Autodesk Inventor part; units mm, degrees
ref_plane "YZ Plane" through (0, 0, 0) normal (1, 0, 0) x (0, 1, 0)
ref_plane "XZ Plane" through (0, 0, 0) normal (0, 1, 0) x (-1, 0, 0)
ref_plane "XY Plane" through (0, 0, 0) normal (0, 0, 1) x (1, 0, 0)
sketch "Sketch1" plane through (0, 0, 0) normal (0, 1, 0) x (-1, 0, 0)
  line L0 (-175, 175) -> (-175, -175)
  line L1 (-175, -175) -> (175, -175)
  line L2 (175, -175) -> (175, 175)
  line L3 (175, 175) -> (-175, 175)
  line L4 (-175, 175) -> (175, -175) construction
  line L5 (-175, -175) -> (175, 175) construction
  point P0 (0, 0)
  dimension "d0" = 350
  dimension "d1" = 350
extrude "Extrusion1" add sketch "Sketch1" along normal blind 10
sketch "Sketch2" plane through (0, 10, 0) normal (0, 1, 0) x (1, 0, 0)
  line L0 (175, -175) -> (175, 175)
  line L1 (175, 175) -> (-175, 175)
  line L2 (-175, 175) -> (-175, -175)
  line L3 (-175, -175) -> (175, -175)
  line L4 (-175, 175) -> (175, -175) construction
  line L5 (-175, -175) -> (175, -175) construction
  line L6 (-175, -175) -> (161.7326, 161.7326) construction
  line L7 (40, -40) -> (40, 40)
  line L8 (40, 40) -> (-40, 40)
  line L9 (-40, 40) -> (-40, -40)
  line L10 (-40, -40) -> (40, -40)
  line L11 (40, -40) -> (-40, 40) construction
  line L12 (40, 40) -> (-40, -40) construction
  point P0 (0, 0)
  dimension "d4" = 80
  dimension "d5" = 80
extrude "Extrusion2" cut sketch "Sketch2" against normal blind 10 contours L10 L9 L8 L7
sketch "Sketch3" plane through (0, 10, 0) normal (0, 1, 0) x (1, 0, 0)
  line L0 (40, -40) -> (-40, -40)
  point P0 (0, 0)
sketch "Sketch4" plane through (0, 10, 0) normal (0, 1, 0) x (1, 0, 0)
  line L0 (40, -40) -> (-40, -40) construction
  line L1 (45, -40) -> (50, -40) construction
  line L2 (45, -40) -> (50, -40)
  line L3 (50, -40) -> (50, -50)
  line L4 (50, -50) -> (40, -50)
  line L5 (40, 40) -> (40, -40)
  line L6 (40, -50) -> (40, -45)
  line L7 (45, -45) -> (40, -45)
  line L8 (45, -45) -> (45, -40)
  line L9 (111.0748, 0) -> (-96.7509, 0) construction
  line L10 (0, -82.157) -> (0, 67.3265) construction
  line L11 (45, 40) -> (50, 40)
  line L12 (50, 40) -> (50, 50)
  line L13 (50, 50) -> (40, 50)
  line L14 (40, 50) -> (40, 45)
  line L15 (45, 45) -> (40, 45)
  line L16 (45, 45) -> (45, 40)
  line L17 (-45, -40) -> (-50, -40)
  line L18 (-50, -40) -> (-50, -50)
  line L19 (-50, -50) -> (-40, -50)
  line L20 (-40, -50) -> (-40, -45)
  line L21 (-45, -45) -> (-40, -45)
  line L22 (-45, -45) -> (-45, -40)
  line L23 (-50, 40) -> (-50, 50)
  line L24 (-45, 45) -> (-45, 40)
  line L25 (-45, 45) -> (-40, 45)
  line L26 (-40, 50) -> (-40, 45)
  line L27 (-50, 50) -> (-40, 50)
  line L28 (-45, 40) -> (-50, 40)
  point P0 (0, 0)
  dimension "d10" = 10
  dimension "d11" = 10
  dimension "d12" = 10
  dimension "d14" = 5
  dimension "d15" = 5
extrude "Extrusion3" cut sketch "Sketch4" against normal blind 10
sketch "Sketch5" plane through (0, 10, 0) normal (0, 1, 0) x (1, 0, 0)
  line L0 (-45, -45) -> (-40, -45)
  line L1 (40, -45) -> (-40, -45)
  line L2 (-40, -45) -> (-40, -50)
  line L3 (-40, -45) -> (-40, -50)
  line L4 (40, -50) -> (40, -45)
  line L5 (-40, -50) -> (40, -50)
  point P0 (0, 0)
extrude "Extrusion4" cut sketch "Sketch5" against normal blind 5
mirror "Mirror1" about plane through (0, 0, 0) normal (0, 0, 1) of "Extrusion4"
properties part number "Bassic Vehicle Chassis"
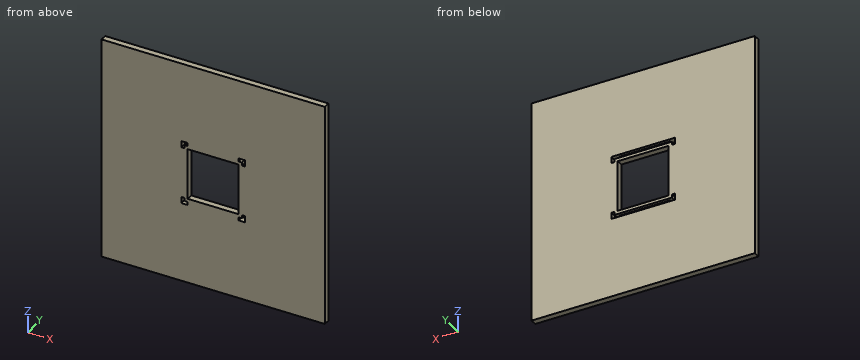
The listing builds one solid part. Answer for the finished solid, in the listing's coordinates (mm). Coordinates: 2 decimals unless noted, no trailing zeros. Write each loop counter-clockwise with the first axis right and the second up, starting at its lowest first coordinate (ties: lowest second). Pieces come first, ordered by that corner, then holes.
Q1. Section B-B, the plane y = 7.5 is taken. Write down the section's boundary in (x, z).
Returned:
outline: (-175, -175) - (175, -175) - (175, 175) - (-175, 175) - close; hole (-50, -50) - (50, -50) - (50, -40) - (45, -40) - (45, -45) - (-45, -45) - (-45, -40) - (-50, -40) - close; hole (-50, 40) - (-45, 40) - (-45, 45) - (45, 45) - (45, 40) - (50, 40) - (50, 50) - (-50, 50) - close; hole (-40, -40) - (40, -40) - (40, 40) - (-40, 40) - close
Q2. Given P1, Ø2.5, axis at x = -11.5, z = 47.5, coming from the +Y side, flat-ended and moving along its own axis, determine where the tip first touches the part or whether it passes through.
Returned:
P1: stops at y = 5
Q3. Section C-C, the plane x = 17 is taken. Write down the section's boundary in (y, z), then the cut area to 3 significant figures.
Returned:
outline: (0, -175) - (10, -175) - (10, -50) - (5, -50) - (5, -45) - (10, -45) - (10, -40) - (0, -40) - close; (0, 40) - (10, 40) - (10, 45) - (5, 45) - (5, 50) - (10, 50) - (10, 175) - (0, 175) - close
area: 2,650 mm2
Q4. Find the intervals of material crossed by line 1 along X through (y, z) = (8, -43.5); line 2 along X through (y, z) = (8.5, 38), in increasing order.
Returned:
line 1: x = -175 to -50, -45 to 45, 50 to 175
line 2: x = -175 to -40, 40 to 175
Q5. Section A-A, the plane z = 13 is taken. Write down the section's boundary in (x, y), then the cut area to 3 significant figures.
Returned:
outline: (-175, 0) - (-40, 0) - (-40, 10) - (-175, 10) - close; (40, 0) - (175, 0) - (175, 10) - (40, 10) - close
area: 2,700 mm2
